Autodesk Inventor part; units mm, degrees
ref_plane "YZ Plane" through (0, 0, 0) normal (1, 0, 0) x (0, 1, 0)
ref_plane "XZ Plane" through (0, 0, 0) normal (0, 1, 0) x (-1, 0, 0)
ref_plane "XY Plane" through (0, 0, 0) normal (0, 0, 1) x (1, 0, 0)
sketch "Skizze2" plane through (0, 0, 0) normal (0, 1, 0) x (-1, 0, 0)
  circle A0 centre (0, 0) radius 2.5
  circle A1 centre (0, 0) radius 2.75
  dimension "d0" = 5
  dimension "d4" = 0.25
extrude "Extrusion1" add sketch "Skizze2" along normal blind 9 contours A0
fillet "Rundung1" radius 2.5 1 edges at (2.5, 9, 0)
extrude "Extrusion2" add sketch "Skizze2" against normal blind 1 contours A0 | A1
properties part number "Head" material "Glas"
Geometry check sheet. Reference: the model listing, model coordinates, mm. A direction names the side the tool comes from. Round coordinates to 2 decimals unless told otherwise and drop trailing zeros. Order: outer loops, then holes, each group sorted by start corner. A loop starts at its lowest first (then second) coordinate and runs counter-clockwise, first axis right, second up. Notation, with made-up numbers: (-18, 23) -> (-5, 23) arc R18 cw to (-5, 27) -> close; hole circle Ø2 at (-10.75, 14.5). An arc over 180 degrees is marked (long way). Return JSON: item names as keys, results as strings. Group by question number.
Q1. Section check A-A, the plane z = 0. Record the boundary of the cut face in (x, y), plus the area to 3 significant figures.
Q2. Material ranges on probe 1 along Y at (x, z) = (1.8, -1.9); probe 2 along Z at (x, y) = (2.3, 1.75); probe 3 along Z at (x, y) = (0.2, 1), recorded low to high. Write a range as from..to.
Q3. Section check C-C, the plane y = 3. Record the boundary of the cut face in (x, z).
Q4. Section check B-B, the plane x = 0. Record the boundary of the cut face in (y, z).
Q5. Tool access check on faces 1 (the cylindrical face through (0.54, 3.2, 2.44)), 2 (the flat face through (0, -1, 0)). Record the directions out of +Z, -Z, +X, -X, +Y, -Y that give a thin tool (end or side, any length) a straight path to the whole face; none if there is none.
Q6. Section check D-D, the plane y = 7.75. Record the boundary of the cut face in (x, z).
Q7. Gauge pin test, flat ends, axial feed: pin 1 (1 mm diameter, centred on x = 1.5, y = 7.5, fed in from -Z); pin 2 (2 mm diameter, centred on x = 2, y = 8, fed in from +Z); pin 3 (1.5 mm diameter, centred on x = 0.5, y = 0.5, fed in from +Z); pin 4 (2 mm diameter, centred on x = -0.5, z = 1, fed in from +Y). Record the tip position at first contact, or that the pin passes through.
Numbers:
{
 "1": {"outline": "(-2.75, -1) -> (2.75, -1) -> (2.75, 0) -> (2.5, 0) -> (2.5, 6.5) arc R2.5 ccw to (-2.5, 6.5) -> (-2.5, 0) -> (-2.75, 0) -> close", "area": "47.8 mm^2"},
 "2": {"probe 1": "-1..0", "probe 2": "-0.98..0.98", "probe 3": "-2.49..2.49"},
 "3": {"outline": "circle Ø5 at (0, 0)"},
 "4": {"outline": "(-1, -2.75) -> (0, -2.75) -> (0, -2.5) -> (6.5, -2.5) arc R2.5 ccw to (6.5, 2.5) -> (0, 2.5) -> (0, 2.75) -> (-1, 2.75) -> close"},
 "5": {"face 1": "+Y", "face 2": "+Z, -Z, +X, -X, -Y"},
 "6": {"outline": "circle Ø4.33 at (0, 0)"},
 "7": {"pin 1": "z = -2.13", "pin 2": "z = 2", "pin 3": "z = 2.75", "pin 4": "y = 9"}
}
